Read the model definition and answer for the solid it produces. Units are mm, in the model's axes. A direction names the side the tool comes from. Coordinates: 2 decimals unless noted, no trailing zeros. Write each loop counter-clockwise with the first axis right and the second up, starting at its lowest first coordinate (ties: lowest second). Pieces come first, ordered by that corner, then holes. Notation, with made-up numbers: (48, 12.5) -> (62, 12.5) arc R24 cw to (62, 43.5) -> close; hole circle Ø7 at (46.5, 56.5). An arc over 180 degrees is marked (long way). One line per item, written item: value. Start each with the question number.
1. Find section A-A, the plane x = -5.09. Write down the section's boundary in (y, z), and give its area (3 significant figures).
2. For a pull along X with two mould halves and no side action, classify faces 1 (the flat face through (-14, 3.48, -16)), 2 (the conical face through (-6.14, 1.875, -10.641)), 3 (the cylindrical face through (-10.588, 2.615, -13.092)) as pulls with the +X half, pulls with the -X half, needs draft (parallel to the pull), parting line crosses it, or undercut.
3. Find section B-B, the plane y = 1.25. Write down the section's boundary in (x, z).
4. For faces 4 (the flat face through (-4.4, 1, -17)), 5 (the flat face through (-12.09, 2.79, -8.99)), determine the directions among +Z, -Z, +X, -X, +Y, -Y from which every point of the face is accessible in a straight line to the end or side of a thin tool.
5. Given P1, Ø1.7, axis at x = -1.5, y = 0.5, coming from the -Z side; P2, Ø1, axis at y = 1.5, z = -16, coming from the +X side; P3, Ø2, axis at x = -8.5, z = -4.5, coming from the +Y side, each flat-ended and moving along its own axis, determine where each tip first touches the part or whether it passes through.
6. Find section D-D, the plane x = -9. Write down the section's boundary in (y, z), and give its area (3 significant figures).
7. Consider line 1 along Y through (x, z) = (-3.5, -4.5); line 2 along X through (y, z) = (1.55, -11); line 3 along Z through (x, y) = (-5.25, 1.3). Determine where each line is inside the solid, lowest interval first.
8. Find section C-C, the plane z = -4.5. Write down the section's boundary in (x, y).
```python
from build123d import *

# Parameters (mm, degrees)
SKETCH1_R           = 1.631999871
BOSS_EXTRUDE1_DEPTH = 2.08
BOSS_EXTRUDE2_DEPTH = 1.4
CHAMFER1_SIZE       = 9
CHAMFER1_SIZE_2     = 1.4
CHAMFER2_SIZE       = 2
CHAMFER2_SIZE2      = 1.5


with BuildPart() as part:
    # Sketch1 → Boss-Extrude1 (new body)
    with BuildSketch(Plane(origin=(0, 0, 0), x_dir=(1, 0, 0), z_dir=(0, 1, 0))):
        with BuildLine():
            Line((-4.4, 14.65), (-4.4, 18.8))
            Line((-4.4, 18.8), (-16.5, 18.8))
            ThreePointArc((-16.5, 18.8), (-13.76109752, 9.4), (-16.5, 0))
            Line((-16.5, 0), (0, 0))
            Line((0, 0), (0, 14.65))
            Line((0, 14.65), (-4.4, 14.65))
        make_face()
        with Locations(Location((-5.09, 9.271001493, 0), (0, 0, 270))):
            Circle(SKETCH1_R, mode=Mode.SUBTRACT)
    extrude(amount=BOSS_EXTRUDE1_DEPTH)

    # Sketch2 → Boss-Extrude2 (add)
    with BuildSketch(Plane(origin=(0, 2.08, 0), x_dir=(1, 0, 0), z_dir=(0, 1, 0))):
        with BuildLine():
            Line((-12.482386169, 18.8), (-16.5, 18.8))
            ThreePointArc((-16.5, 18.8), (-13.964523784, 12.06055201), (-14.35739556, 4.870666711))
            Line((-14.35739556, 4.870666711), (-10.976655168, 3.964800053))
            ThreePointArc((-10.976655168, 3.964800053), (-10.36843652, 11.520546233), (-12.482386169, 18.8))
        make_face()
    extrude(amount=BOSS_EXTRUDE2_DEPTH)

    # Chamfer1
    # the kernel refuses this chamfer: 9, 1.4 mm, written as the material it takes off along each edge
    with BuildSketch(Plane(origin=(-36.950124299, 3.48, -10.924370131), x_dir=(0.25881451828946306, 0.005914407767472668, -0.9659089319927389), z_dir=(0.9659258262890682, 0, 0.2588190451025212))) as chamfer1_piece_1_section:
        Polygon((CHAMFER1_SIZE * 0.999982509737, -CHAMFER1_SIZE * 0.00591440776747), (-CHAMFER1_SIZE_2 * 0.00591440776747, -CHAMFER1_SIZE_2 * 0.999982509737), (0, 0), align=None)
    chamfer1_piece_1 = extrude(amount=50.279427829, mode=Mode.PRIVATE)
    chamfer1_piece_1 = split(chamfer1_piece_1, bisect_by=Plane(origin=(-11.82064593, 2.08, -7.576464434), z_dir=(0, 1, 0)), keep=Keep.TOP, mode=Mode.PRIVATE)
    add(chamfer1_piece_1, mode=Mode.SUBTRACT)

    # Chamfer2
    chamfer2_edges = [part.edges().sort_by_distance(p)[0] for p in [
        (-5.09, 0, -10.903001364),
    ]]
    chamfer2_side = [part.faces().sort_by_distance(p)[0] for p in [
        (-5.09, 1.04, -10.903001364),
    ]]
    chamfer(chamfer2_edges, length=CHAMFER2_SIZE, length2=CHAMFER2_SIZE2, reference=chamfer2_side[0])


solid = part.part
```
Answer block:
1. outline: (0, -18.8) -> (2.08, -18.8) -> (2.08, -10.9) -> (2, -10.9) -> (0, -12.4) -> close; (0, -6.14) -> (2, -7.64) -> (2.08, -7.64) -> (2.08, 0) -> (0, 0) -> close
1. area: 29.3 mm2
2. face 1: needs draft
2. face 2: undercut
2. face 3: pulls with the +X half
3. outline: (-16.5, -18.8) -> (-4.4, -18.8) -> (-4.4, -14.65) -> (0, -14.65) -> (0, 0) -> (-16.5, 0) arc R17.5 cw to start; hole circle Ø4.39 at (-5.09, -9.27)
4. face 4: -Z, +X, +Y, -Y
4. face 5: +Z, -X, +Y
5. P1: stops at z = -14.65
5. P2: stops at x = -4.4
5. P3: stops at y = 2.08
6. outline: (0, -18.8) -> (2.08, -18.8) -> (2.08, 0) -> (0, 0) -> close
6. area: 39.1 mm2
7. line 1: y = 0 to 2.08
7. line 2: x = -13.83 to -6.03, -4.15 to 0
7. line 3: z = -18.8 to -11.42, -7.12 to 0
8. outline: (-14.46, 0) -> (0, 0) -> (0, 2.08) -> (-10.84, 2.08) -> (-10.84, 2.17) -> (-12.97, 2.08) -> (-14.46, 2.08) -> close
